Check sheet for the modelled part. Datum: model origin and axes. Units: mm. A direction names the side the tool comes from. Give positions to 0.01 mm unless a question says otherwise; leave off trailing zeros. Write each loop counter-clockwise with the first axis right and the second up, starting at its lowest first coordinate (ties: lowest second). Pieces come first, ordered by that corner, then holes. Notation, with made-up numbers: (32.25, 63) -> (62.25, 63) arc R20 ccw to (62.25, 100) -> close; hole circle Ø11 at (-37, -17.5). An arc over 180 degrees is marked (long way). Use a Markdown table: item, result. Add a question column.
1. Cross-section at B-B (y = 0). Enter the section's corners in (x, z).
2. Cross-section at D-D (x = -39). Enter the section's corners in (y, z), then the cut area to 3 significant figures.
3. Scan lines: probe 1 along Y at (x, z) = (0, 5.75); probe 2 along Y at (x, z) = (43.5, 13); probe 3 along Y at (x, z) = (36.5, 9.25). Record each from-to range of solid material in increasing order. Write a range as [from, to].
4. Cross-section at C-C (z = 12). Enter the section's corners in (x, y).
5. Release check for a two-part mould opening along X. For faces 3 (the cylindrical face through (11.535, 3.633, 9.266)), 4 (the cylindrical face through (88.744, 25.155, 9.266)), 5 (the flat face through (0, -16, 18.796)) record: released by +X, released by -X, zero draft, split by the parting line, or undercut.
6. Gauge pin test, flat ends, axial feed: P1, Ø5, axis at y = -21.5, z = 10, coming from the -X side; P2, Ø6, axis at x = 69, z = 16.5, coming from the +Y side; P3, Ø5.5, axis at x = 45.5, z = 11.5, coming from the +Y side. Record the tip position at first contact, or that the pin passes through.
7. Cross-section at A-A (x = 0). Enter the section's corners in (y, z).
8. Set-up check for faces 1 (the flat face through (0, -16, 0)), 2 (the flat face through (-54, -6.179, 9)): record each of +Z, -Z, +X, -X, +Y, -Y from which the full face is reachable in a straight line by a thin tool's end or side.
from build123d import *

# Parameters (mm, degrees)
F0_R     = 93.0402692982
F0_R_2   = 20.2691960741
F0_R_3   = 12.0935741479
F1_DEPTH = 18.796


with BuildPart() as f1:
    # F0 (on Top) → F1 (new body)
    with BuildSketch(Plane.XY):
        with Locations((0, -2.7915611863)):
            Circle(F0_R)
        with BuildLine():
            ThreePointArc((-79.8869530557, 13.3503982046), (-0.497116202, 80.9932792041), (79.7170577495, 14.3300071359))
            ThreePointArc((79.7170577495, 14.3300071359), (80.674735607, 7.1934300229), (80.9948047763, 0))
            ThreePointArc((80.9948047763, 0), (80.9212005693, -3.4522020762), (80.7005217242, -6.8981297599))
            ThreePointArc((80.7005217242, -6.8981297599), (-0.3608473211, -80.9940009504), (-80.7587824796, -6.1787905904))
            ThreePointArc((-80.7587824796, -6.1787905904), (-80.9142162427, 3.6122030091), (-79.8869530557, 13.3503982046))
        make_face(mode=Mode.SUBTRACT)
        with BuildLine():
            ThreePointArc((25.7351095282, -6.8981297599), (26.4154818423, -3.4788468851), (26.6435743963, 0))
            ThreePointArc((26.6435743963, 0), (25.576764867, 7.4638566138), (22.461766451, 14.3300071359))
            ThreePointArc((22.461766451, 14.3300071359), (-0.5732574504, 26.6374066401), (-23.0574700345, 13.3503982046))
            ThreePointArc((-23.0574700345, 13.3503982046), (-26.362426228, 3.8603808085), (-25.9172259984, -6.1787905904))
            ThreePointArc((-25.9172259984, -6.1787905904), (-0.371017267, -26.6409910251), (25.7351095282, -6.8981297599))
        make_face()
        Circle(F0_R_2, mode=Mode.SUBTRACT)
        Circle(F0_R_2)
        Circle(F0_R_3, mode=Mode.SUBTRACT)
        with BuildLine():
            ThreePointArc((22.461766451, 14.3300071359), (25.576764867, 7.4638566138), (26.6435743963, 0))
            ThreePointArc((26.6435743963, 0), (26.4154818423, -3.4788468851), (25.7351095282, -6.8981297599))
            Line((25.7351095282, -6.8981297599), (80.7005217242, -6.8981297599))
            ThreePointArc((80.7005217242, -6.8981297599), (80.9212005693, -3.4522020762), (80.9948047763, 0))
            ThreePointArc((80.9948047763, 0), (80.674735607, 7.1934300229), (79.7170577495, 14.3300071359))
            Line((79.7170577495, 14.3300071359), (22.461766451, 14.3300071359))
        make_face()
        with BuildLine():
            ThreePointArc((-25.9172259984, -6.1787905904), (-26.362426228, 3.8603808085), (-23.0574700345, 13.3503982046))
            Line((-23.0574700345, 13.3503982046), (-79.8869530557, 13.3503982046))
            ThreePointArc((-79.8869530557, 13.3503982046), (-80.9142162427, 3.6122030091), (-80.7587824796, -6.1787905904))
            Line((-80.7587824796, -6.1787905904), (-25.9172259984, -6.1787905904))
        make_face()
    extrude(amount=F1_DEPTH)


solid = f1.part
Worked answers:
| question | item | result |
|---|---|---|
| 1 | outline | (-93, 0) -> (-12.09, 0) -> (-12.09, 18.8) -> (-93, 18.8) -> close; (12.09, 0) -> (93, 0) -> (93, 18.8) -> (12.09, 18.8) -> close |
| 2 | outline | (-87.26, 0) -> (-70.99, 0) -> (-70.99, 18.8) -> (-87.26, 18.8) -> close; (-6.18, 0) -> (13.35, 0) -> (13.35, 18.8) -> (-6.18, 18.8) -> close; (70.99, 0) -> (81.68, 0) -> (81.68, 18.8) -> (70.99, 18.8) -> close |
| 2 | area | 874 mm² |
| 3 | probe 1 | y = [-95.83, -80.99], [-26.64, -12.09], [12.09, 26.64], [80.99, 90.25] |
| 3 | probe 2 | y = [-85.04, -68.32], [-6.9, 14.33], [68.32, 79.45] |
| 3 | probe 3 | y = [-88.37, -72.3], [-6.9, 14.33], [72.3, 82.79] |
| 4 | outline | circle Ø186.08 at (0, -2.79); hole (-80.76, -6.18) arc R80.99 ccw to (80.7, -6.9) -> (25.74, -6.9) arc R26.64 cw to (-25.92, -6.18) -> close; hole (-79.89, 13.35) -> (-23.06, 13.35) arc R26.64 cw to (22.46, 14.33) -> (79.72, 14.33) arc R80.99 ccw to start; hole circle Ø24.19 at (0, 0) |
| 5 | face 3 | undercut |
| 5 | face 4 | split by the parting line |
| 5 | face 5 | zero draft |
| 6 | P1 | stops at x = -91.62 |
| 6 | P2 | stops at y = 62.79 |
| 6 | P3 | stops at y = 79.85 |
| 7 | outline | (-95.83, 0) -> (-80.99, 0) -> (-80.99, 18.8) -> (-95.83, 18.8) -> close; (-26.64, 0) -> (-12.09, 0) -> (-12.09, 18.8) -> (-26.64, 18.8) -> close; (12.09, 0) -> (26.64, 0) -> (26.64, 18.8) -> (12.09, 18.8) -> close; (80.99, 0) -> (90.25, 0) -> (90.25, 18.8) -> (80.99, 18.8) -> close |
| 8 | face 1 | -Z, +X, -X, +Y, -Y |
| 8 | face 2 | +Z, -Z |
